```python
from build123d import *

# Parameters (mm, degrees)
SKETCH1_R           = 3.2639
BOSS_EXTRUDE1_DEPTH = 1.524


with BuildPart() as part:
    # Sketch1 → Boss-Extrude1 (new body)
    with BuildSketch(Plane.XY):
        with BuildLine():
            Line((0, 0), (0, 25.4))
            ThreePointArc((0, 25.4), (7.9375, 33.3375), (15.875, 25.4))
            Line((15.875, 25.4), (15.875, 0))
            Line((15.875, 0), (0, 0))
        make_face()
        with Locations(Location((7.9375, 25.4, 0), (0, 0, 180))):
            Circle(SKETCH1_R, mode=Mode.SUBTRACT)
    extrude(amount=BOSS_EXTRUDE1_DEPTH)


solid = part.part
```
Could you check a few things on this model? Use its own coordinates, in mm. Coordinates: 2 decimals unless noted, no trailing zeros. Order: outer loops, then holes, each group sorted by start corner. A loop starts at its lowest first (then second) coordinate and runs counter-clockwise, first axis right, second up. Notation, with made-up numbers: M -10.5,58.25 L 41.5,58.25 A18 cw 41.5,84.25 Z; hole C 8,34 d6. An arc over 180 degrees is marked long. Use one line per item in the form item = value. Start each with the question number.
1. Please list where these lines run through material, in increasing order: line 1 (X direction, y = 25.4, z = 0.85) (3 decimals); line 2 (X direction, y = 23, z = 0.8) (3 decimals); line 3 (Y direction, x = 7.5, z = 0.3).
2. Suppose I cut it at C-C on x = 10. Write out the boundary of the cut face in (y, z).
3. Suppose I cut it at D-D on y = 30. Write out the boundary of the cut face in (x, z), then the cut area to 3 significant figures.
4. For pin 1 (3 mm diameter, centred on x = 13, y = 13, fed in from -Z), with a flat end and sliding along its axis, tell me the tip position at first contact or that it passes through.
5. Suppose I cut it at A-A on y = 26.5. Write out the boundary of the cut face in (x, z), then the cut area to 3 significant figures.
6. We'd pull the mould along Y, two halves only. Please class faces 1 (the flat face through (8, 17, 0)), 2 (the cylindrical face through (7.763, 33.336, 0.751)), 3 (the cylindrical face through (8.362, 22.164, 0.751)): +Y half, -Y half, draft (parallel to the pull), parting line (faces both ways), or undercut.
7. Suppose I cut it at B-B on z = 1.25. Write out the boundary of the cut face in (x, y) (1 decimal), then the cut area to 3 significant figures.
Geometry says:
q1.line_1 = 0 to 4.674, 11.201 to 15.875
q1.line_2 = 0 to 5.725, 10.15 to 15.875
q1.line_3 = 0 to 22.17, 28.63 to 33.33
q2.outline = M 0,0 L 22.87,0 L 22.87,1.52 L 0,1.52 Z; M 27.93,0 L 33.06,0 L 33.06,1.52 L 27.93,1.52 Z
q3.outline = M 1.47,0 L 14.41,0 L 14.41,1.52 L 1.47,1.52 Z
q3.area = 19.7 mm^2
q4.pin_1 = 0
q5.outline = M 0.08,0 L 4.86,0 L 4.86,1.52 L 0.08,1.52 Z; M 11.01,0 L 15.8,0 L 15.8,1.52 L 11.01,1.52 Z
q5.area = 14.6 mm^2
q6.face_1 = draft
q6.face_2 = +Y half
q6.face_3 = undercut
q7.outline = M 0,0 L 15.9,0 L 15.9,25.4 A7.9 ccw 0,25.4 Z; hole C 7.9,25.4 d6.5
q7.area = 469 mm^2
